```python
from build123d import *

# Parameters (mm, degrees)
SKETCH_2_R           = 10.01
SKETCH_2_R_2         = 9
EXTRUDE_2_DEPTH      = 25
EXTRUDE_START        = 2
SKETCH_3_R           = 10.01
EXTRUDE_3_DEPTH      = 2
SKETCH_4_R           = 9
CUT_EXTRUDE_1_DEPTH  = 1
SKETCH_6_R           = 8
CUT_EXTRUDE_3_DEPTH  = 3
SKETCH_7_R           = 11
SKETCH_7_R_2         = 10
EXTRUDE_4_DEPTH      = 4
SKETCH_8_R           = 9
SKETCH_8_R_2         = 8
EXTRUDE_5_DEPTH      = 25
SKETCH_10_R          = 10.01
SKETCH_10_R_2        = 9.5
CUT_EXTRUDE_5_DEPTH  = 1
CUT_EXTRUDE_START    = 10
SKETCH_11_R          = 10.01
CUT_EXTRUDE_6_DEPTH  = 10
SKETCH_12_R          = 11
SKETCH_12_R_2        = 10.01
EXTRUDE_6_DEPTH      = 26
SKETCH_13_R          = 9
CUT_EXTRUDE_7_DEPTH  = 26
SKETCH_14_R          = 10.005206388
SKETCH_14_R_2        = 9.5
EXTRUDE_7_DEPTH      = 26
SKETCH_16_R          = 11
SKETCH_16_R_2        = 10.5
CUT_EXTRUDE_12_DEPTH = 1
SKETCH_17_R          = 13.732639959
CUT_EXTRUDE_13_DEPTH = 1
SKETCH_19_R          = 10.229377856
SKETCH_19_R_2        = 10.005206388
EXTRUDE_10_DEPTH     = 10
SKETCH_20_R          = 12
SKETCH_20_R_2        = 11
EXTRUDE_11_DEPTH     = 2


with BuildPart() as part:
    # Sketch 2 → Extrude 2 (new body)
    with BuildSketch(Plane.XZ):
        with Locations(Location((0, 0, 0), (0, 0, 270))):
            Circle(SKETCH_2_R)
        with Locations(Location((0, 0, 0), (0, 0, 270))):
            Circle(SKETCH_2_R_2, mode=Mode.SUBTRACT)
    extrude(amount=EXTRUDE_2_DEPTH)

    # Sketch 3 → Extrude 3 (add)
    with BuildSketch(Plane(origin=(0, 0, 0), x_dir=(1, 0, 0), z_dir=(0, 1, 0)).offset(EXTRUDE_START)):
        with Locations(Location((0, 0, 0), (0, 0, 270))):
            Circle(SKETCH_3_R)
    extrude(amount=-EXTRUDE_3_DEPTH)

    # Sketch 4 → Cut-Extrude 1 (cut)
    with BuildSketch(Plane(origin=(0, 2, 0), x_dir=(1, 0, 0), z_dir=(0, 1, 0))):
        with Locations(Location((0, 0, 0), (0, 0, 90))):
            Circle(SKETCH_4_R)
    extrude(amount=-CUT_EXTRUDE_1_DEPTH, mode=Mode.SUBTRACT)

    # Sketch 6 → Cut-Extrude 3 (cut)
    with BuildSketch(Plane(origin=(0, 1, 0), x_dir=(1, 0, 0), z_dir=(0, 1, 0))):
        with Locations(Location((0, 0, 0), (0, 0, 270))):
            Circle(SKETCH_6_R)
    extrude(amount=-CUT_EXTRUDE_3_DEPTH, mode=Mode.SUBTRACT)

    # Sketch 7 → Extrude 4 (add)
    with BuildSketch(Plane(origin=(0, 1, 0), x_dir=(1, 0, 0), z_dir=(0, 1, 0))):
        with Locations(Location((0, 0, 0), (0, 0, 270))):
            Circle(SKETCH_7_R)
        with Locations(Location((0, 0, 0), (0, 0, 270))):
            Circle(SKETCH_7_R_2, mode=Mode.SUBTRACT)
    extrude(amount=EXTRUDE_4_DEPTH)

    # Sketch 8 → Extrude 5 (add)
    with BuildSketch(Plane.XZ):
        with Locations(Location((0, 0, 0), (0, 0, 90))):
            Circle(SKETCH_8_R)
        with Locations(Location((0, 0, 0), (0, 0, 90))):
            Circle(SKETCH_8_R_2, mode=Mode.SUBTRACT)
    extrude(amount=EXTRUDE_5_DEPTH)

    # Sketch 10 → Cut-Extrude 5 (cut)
    with BuildSketch(Plane.XZ.offset(-1)):
        with Locations(Location((0, 0, 0), (0, 0, 270))):
            Circle(SKETCH_10_R)
        with Locations(Location((0, 0, 0), (0, 0, 270))):
            Circle(SKETCH_10_R_2, mode=Mode.SUBTRACT)
    extrude(amount=CUT_EXTRUDE_5_DEPTH, mode=Mode.SUBTRACT)

    # Sketch 11 → Cut-Extrude 6 (cut)
    with BuildSketch(Plane(origin=(0, 1, 0), x_dir=(1, 0, 0), z_dir=(0, 1, 0)).offset(CUT_EXTRUDE_START)):
        with Locations(Location((0, 0, 0), (0, 0, 90))):
            Circle(SKETCH_11_R)
    extrude(amount=-CUT_EXTRUDE_6_DEPTH, mode=Mode.SUBTRACT)


with BuildPart() as cut_extrude_6_piece_1:
    # of the separate pieces the step leaves, piece 1, a body of its own (cut_extrude_6_pieces)
    add(part.part.solids().sort_by_distance((0, 0, -10.01))[0])



with BuildPart() as cut_extrude_6_piece_2:
    # of the separate pieces the step leaves, piece 2, a body of its own (cut_extrude_6_pieces)
    add(part.part.solids().sort_by_distance((0, 1, 11))[0])


with BuildPart() as cut_extrude_6_piece_1_1:
    add(cut_extrude_6_piece_1.part)

    add(cut_extrude_6_piece_2.part)  # Extrude 6 merges Cut-Extrude 6 piece 2
    # Sketch 12 → Extrude 6 (add)
    with BuildSketch(Plane.XZ.offset(25)):
        with Locations(Location((0, 0, 0), (0, 0, 270))):
            Circle(SKETCH_12_R)
        with Locations(Location((0, 0, 0), (0, 0, 270))):
            Circle(SKETCH_12_R_2, mode=Mode.SUBTRACT)
    extrude(amount=-EXTRUDE_6_DEPTH)

    # Sketch 13 → Cut-Extrude 7 (cut)
    with BuildSketch(Plane(origin=(0, 1, 0), x_dir=(1, 0, 0), z_dir=(0, 1, 0))):
        with Locations(Location((0, 0, 0), (0, 0, 270))):
            Circle(SKETCH_13_R)
    extrude(amount=-CUT_EXTRUDE_7_DEPTH, mode=Mode.SUBTRACT)

    # Sketch 14 → Extrude 7 (add)
    with BuildSketch(Plane(origin=(0, 1, 0), x_dir=(1, 0, 0), z_dir=(0, 1, 0))):
        with Locations(Location((0, 0, 0), (0, 0, 270))):
            Circle(SKETCH_14_R)
        Circle(SKETCH_14_R_2, mode=Mode.SUBTRACT)
    extrude(amount=-EXTRUDE_7_DEPTH)

    # Sketch 16 → Cut-Extrude 12 (cut)
    with BuildSketch(Plane.XZ.offset(-2)):
        with Locations(Location((0, 0, 0), (0, 0, 270))):
            Circle(SKETCH_16_R)
        with Locations(Location((0, 0, 0), (0, 0, 270))):
            Circle(SKETCH_16_R_2, mode=Mode.SUBTRACT)
    extrude(amount=CUT_EXTRUDE_12_DEPTH, mode=Mode.SUBTRACT)

    # Sketch 17 → Cut-Extrude 13 (cut)
    with BuildSketch(Plane(origin=(0, 5, 0), x_dir=(1, 0, 0), z_dir=(0, 1, 0))):
        Circle(SKETCH_17_R)
    extrude(amount=-CUT_EXTRUDE_13_DEPTH, mode=Mode.SUBTRACT)

    # Sketch 19 → Extrude 10 (add)
    with BuildSketch(Plane(origin=(0, 1, 0), x_dir=(1, 0, 0), z_dir=(0, 1, 0))):
        Circle(SKETCH_19_R)
        Circle(SKETCH_19_R_2, mode=Mode.SUBTRACT)
    extrude(amount=-EXTRUDE_10_DEPTH)

    # Sketch 20 → Extrude 11 (add)
    with BuildSketch(Plane(origin=(0, 4, 0), x_dir=(1, 0, 0), z_dir=(0, 1, 0))):
        with Locations(Location((0, 0, 0), (0, 0, 270))):
            Circle(SKETCH_20_R)
        with Locations(Location((0, 0, 0), (0, 0, 90))):
            Circle(SKETCH_20_R_2, mode=Mode.SUBTRACT)
    extrude(amount=-EXTRUDE_11_DEPTH)


solid = cut_extrude_6_piece_1_1.part
```
The model under review builds one solid part; all positions refer to its coordinate system, in mm. A direction names the side the tool comes from. Give positions to 0.01 mm unless a question says otherwise; leave off trailing zeros. Write each loop counter-clockwise with the first axis right and the second up, starting at its lowest first coordinate (ties: lowest second). Pieces come first, ordered by that corner, then holes.
(1) The part is to be moulded in two halves that separate along X. For faces 6 (the flat face through (-4, 1, -10)), 7 (the cylindrical face through (2.703, -11.818, 8.584)), 8 (the flat face through (-9, 1, -2)), 9 (the cylindrical face through (3.604, 3.014, 11.446)), say which applies: released by +X, released by -X, zero draft, split by the parting line, or undercut.
(2) For P1, Ø10, axis at y = -11, z = -1, coming from the +X side; P2, Ø1, axis at x = 5, y = -12.5, coming from the +Z side; P3, Ø6, axis at x = -6.5, y = -1, coming from the +Z side, all flat-tipped, find the tip position at first contact; note any pin that passes through.
(3) Consider section B-B, the plane z = 0. Give the boundary of the cut face in (x, y).
(4) Tool access review of faces 1 (the cylindrical face through (-10.74, -12.18, 2.38)), 2 (the cylindrical face through (3.2, 1.5, -10)), 3 (the flat face through (9, -25, 2)), 4 (the flat face through (-10, 4, 3)), 5 (the cylindrical face through (-6.091, 2.479, 7.944)): name each direction out of +Z, -Z, +X, -X, +Y, -Y from which nothing blocks a thin tool from reaching the whole face with its end or side.
(5) Consider section A-A, the plane x = 0. Give the boundary of the cut face in (y, z).
(6) To check wall thickness, follow L1, parallel to X at y = -11.25, z = 0; L2, parallel to X at y = 1.7, z = 0; L3, parallel to Y at x = -4.5, z = 8. State the ranges of each line that lie inside material, in increasing order.
(7) Consider section C-C, the plane y = -10. Give the boundary of the cut face in (x, z).
Returned:
1. face 6: zero draft
1. face 7: undercut
1. face 8: undercut
1. face 9: split by the parting line
2. P1: stops at x = 11
2. P2: stops at z = 10.04
2. P3: stops at z = 10.43
3. outline: (-12, 2) - (-10.5, 2) - (-10.5, 1) - (-11, 1) - (-11, -25) - (-9, -25) - (-9, 1) - (-10.01, 1) - (-10.01, 4) - (-12, 4) - close; (9, -25) - (11, -25) - (11, 1) - (10.5, 1) - (10.5, 2) - (12, 2) - (12, 4) - (10.01, 4) - (10.01, 1) - (9, 1) - close
4. face 1: -Y
4. face 2: none
4. face 3: +Z, -Z, +X, -X, -Y
4. face 4: +Z, -Z, +X, -X, +Y
4. face 5: +Y
5. outline: (-25, -11) - (1, -11) - (1, -10.5) - (2, -10.5) - (2, -12) - (4, -12) - (4, -10.01) - (1, -10.01) - (1, -9) - (-25, -9) - close; (-25, 9) - (1, 9) - (1, 10.01) - (4, 10.01) - (4, 12) - (2, 12) - (2, 10.5) - (1, 10.5) - (1, 11) - (-25, 11) - close
6. L1: x = -11 to -9, 9 to 11
6. L2: x = -10.5 to -10.01, 10.01 to 10.5
6. L3: y = -25 to 1
7. outline: circle Ø22 at (0, 0); hole circle Ø18 at (0, 0)
